```python
from build123d import *

# Parameters (mm, degrees)
SKETCH1_R           = 1.7
BOSS_EXTRUDE1_DEPTH = 6.35


with BuildPart() as part:
    # Sketch1 → Boss-Extrude1 (new body)
    with BuildSketch(Plane(origin=(0, 0, 0), x_dir=(1, 0, 0), z_dir=(0, 1, 0))):
        with BuildLine():
            Line((-131.683125, 82.55), (-131.683125, 44.45))
            Line((-131.683125, 44.45), (-125.333125, 44.45))
            Line((-125.333125, 44.45), (-125.333125, 69.85))
            Line((-125.333125, 69.85), (-77.073125, 69.85))
            Line((-77.073125, 69.85), (-77.073125, 44.45))
            Line((-77.073125, 44.45), (-70.723125, 44.45))
            Line((-70.723125, 44.45), (-70.723125, 69.85))
            Line((-70.723125, 69.85), (-22.463125, 69.85))
            Line((-22.463125, 69.85), (-22.463125, 44.45))
            Line((-22.463125, 44.45), (-16.113125, 44.45))
            Line((-16.113125, 44.45), (-16.113125, 69.85))
            Line((-16.113125, 69.85), (32.146875, 69.85))
            Line((32.146875, 69.85), (32.146875, 44.45))
            Line((32.146875, 44.45), (38.496875, 44.45))
            Line((38.496875, 44.45), (38.496875, 69.85))
            Line((38.496875, 69.85), (86.756875, 69.85))
            Line((86.756875, 69.85), (86.756875, 44.45))
            Line((86.756875, 44.45), (93.106875, 44.45))
            Line((93.106875, 44.45), (93.106875, 82.55))
            ThreePointArc((93.106875, 82.55), (91.247003061, 87.040128061), (86.756875, 88.9))
            Line((86.756875, 88.9), (-125.333125, 88.9))
            ThreePointArc((-125.333125, 88.9), (-129.823253061, 87.040128061), (-131.683125, 82.55))
        make_face()
        with Locations(Location((-86.756875, 79.375, 0), (0, 0, 270))):
            Circle(SKETCH1_R, mode=Mode.SUBTRACT)
        with Locations(Location((-19.288125, 79.375, 0), (0, 0, 270))):
            Circle(SKETCH1_R, mode=Mode.SUBTRACT)
        with Locations(Location((48.180625, 79.375, 0), (0, 0, 270))):
            Circle(SKETCH1_R, mode=Mode.SUBTRACT)
    extrude(amount=BOSS_EXTRUDE1_DEPTH)


solid = part.part
```
Geometry check sheet. Reference: the model listing, model coordinates, mm. A direction names the side the tool comes from. Round coordinates to 2 decimals unless told otherwise and drop trailing zeros. Loops run counter-clockwise (first coordinate to the right, second up) from the corner with the lowest first, then second, coordinate; pieces in that order, holes last. Notation, with made-up numbers: M 11.5,-27 L 62.5,-27 A34 ccw 62.5,5 Z; hole C 30,59.25 d9. An arc over 180 degrees is marked long. Return JSON: item names as keys, results as strings. Group by question number.
(1) Section check B-B, the plane y = 3.5. Enter the section's corners in (x, z) (3 decimals), and give its area (3 significant figures).
(2) Set-up check for faces 5 (the face through (-70.723, 3, -57)), 6 (the face through (-129, 3, -44.45)): record each of +Z, -Z, +X, -X, +Y, -Y from which the full face is reachable in a straight line by a thin tool's end or side.
(3) Section check C-C, the plane x = 43. Enter the section's corners in (y, z).
(4) Section check A-A, the plane z = -62.5. Enter the section's corners in (x, y), and give its area (3 significant figures).
(5) Scan lines: line 1 along X through (y, z) = (2.5, -58.5); line 2 along Z through (x, y) = (68.5, 3.75); line 3 along X through (y, z) = (5.75, -83). Record each from-to range of solid material in increasing order. Write a range as [from, to].
(6) Go/stop test with flat-tipped pins: pin 1 (2.5 mm diameter, centred on x = -19.29, z = -79.38, fed in from -Y); pin 2 (1.9 mm diameter, centred on x = 18, y = 4.5, fed in from +Z). Record where each tip stops, or that it passes through.
(7) Mould release check, pull along X, two halves, no side actions. Record for faces 1 (the face through (91.296, 3.131, -86.99)), 2 (the face through (-22.463, 3, -57)), 3 (the face through (-18, 3, -88.9)), 4 (the face through (-125.333, 3, -57)): pulls with the +X half, pulls with the -X half, needs draft (parallel to the pull), parting line crosses it, or undercut.
Data:
{
 "1": {"outline": "M -131.683,-82.55 A6.35 ccw -125.333,-88.9 L 86.757,-88.9 A6.35 ccw 93.107,-82.55 L 93.107,-44.45 L 86.757,-44.45 L 86.757,-69.85 L 38.497,-69.85 L 38.497,-44.45 L 32.147,-44.45 L 32.147,-69.85 L -16.113,-69.85 L -16.113,-44.45 L -22.463,-44.45 L -22.463,-69.85 L -70.723,-69.85 L -70.723,-44.45 L -77.073,-44.45 L -77.073,-69.85 L -125.333,-69.85 L -125.333,-44.45 L -131.683,-44.45 Z; hole C -86.757,-79.375 d3.4; hole C -19.288,-79.375 d3.4; hole C 48.181,-79.375 d3.4", "area": "5,040 mm²"},
 "2": {"face 5": "+Z, +Y, -Y", "face 6": "+Z, +X, -X, +Y, -Y"},
 "3": {"outline": "M 0,-88.9 L 6.35,-88.9 L 6.35,-69.85 L 0,-69.85 Z"},
 "4": {"outline": "M -131.68,0 L -125.33,0 L -125.33,6.35 L -131.68,6.35 Z; M -77.07,0 L -70.72,0 L -70.72,6.35 L -77.07,6.35 Z; M -22.46,0 L -16.11,0 L -16.11,6.35 L -22.46,6.35 Z; M 32.15,0 L 38.5,0 L 38.5,6.35 L 32.15,6.35 Z; M 86.76,0 L 93.11,0 L 93.11,6.35 L 86.76,6.35 Z", "area": "202 mm²"},
 "5": {"line 1": "[-131.68, -125.33], [-77.07, -70.72], [-22.46, -16.11], [32.15, 38.5], [86.76, 93.11]", "line 2": "[-88.9, -69.85]", "line 3": "[-131.67, 93.09]"},
 "6": {"pin 1": "through", "pin 2": "z = -69.85"},
 "7": {"face 1": "pulls with the +X half", "face 2": "undercut", "face 3": "needs draft", "face 4": "undercut"}
}
